from build123d import *

# Parameters (mm, degrees)
SKETCH3_W                = 76.2
SKETCH3_H                = 25.4
SKETCH3_R                = 3.175
BOSS_EXTRUDE1_DEPTH      = 2.286
BOSS_EXTRUDE1_DEPTH_BACK = 2.286


with BuildPart() as part:
    # Sketch3 → Boss-Extrude1 (new body, two sides)
    with BuildSketch(Plane.XY) as boss_extrude1_sk:
        Rectangle(SKETCH3_W, SKETCH3_H)
        with Locations((-28.575, 0)):
            Circle(SKETCH3_R, mode=Mode.SUBTRACT)
        with Locations((28.575, 0)):
            Circle(SKETCH3_R, mode=Mode.SUBTRACT)
    extrude(amount=BOSS_EXTRUDE1_DEPTH)
    extrude(boss_extrude1_sk.sketch, amount=-BOSS_EXTRUDE1_DEPTH_BACK)


solid = part.part
CAD build for the part. Positions are in the model's coordinates, mm. Round coordinates to 2 decimals unless told otherwise and drop trailing zeros. Loops run counter-clockwise (first coordinate to the right, second up) from the corner with the lowest first, then second, coordinate; pieces in that order, holes last. Notation, with made-up numbers: (18, -8.75) - (38, -8.75) arc R27 ccw to (38, 21.25) - close; hole circle Ø6 at (22.5, 38). An arc over 180 degrees is marked (long way). Put each result on its own line as item: value.
1. Two-plate mould, pull along X, no slides. Class faces 1 (the flat face through (-1, 12.7, 0)), 2 (the cylindrical face through (-31.095, -1.932, -0.032)), 3 (the flat face through (38.1, 0, 0)), 4 (the cylindrical face through (25.4, 0.1, 0)): released by +X, released by -X, zero draft, split by the parting line, or undercut.
Geometry check:
face 1: zero draft
face 2: undercut
face 3: released by +X
face 4: undercut
2. Slice it at B-B on x = 29.5. List the corners of the cut face in (y, z), and give its area (3 significant figures).
Geometry check:
outline: (-12.7, -2.29) - (-3.04, -2.29) - (-3.04, 2.29) - (-12.7, 2.29) - close; (3.04, -2.29) - (12.7, -2.29) - (12.7, 2.29) - (3.04, 2.29) - close
area: 88.4 mm²
3. Slice it at C-C on z = 0.8. List the corners of the cut face in (x, y) (3 decimals).
Geometry check:
outline: (-38.1, -12.7) - (38.1, -12.7) - (38.1, 12.7) - (-38.1, 12.7) - close; hole circle Ø6.35 at (-28.575, 0); hole circle Ø6.35 at (28.575, 0)
4. Slice it at D-D on x = -30. List the corners of the cut face in (y, z).
Geometry check:
outline: (-12.7, -2.29) - (-2.84, -2.29) - (-2.84, 2.29) - (-12.7, 2.29) - close; (2.84, -2.29) - (12.7, -2.29) - (12.7, 2.29) - (2.84, 2.29) - close
5. Slice it at A-A on y = 0. List the corners of the cut face in (x, z).
Geometry check:
outline: (-38.1, -2.29) - (-31.75, -2.29) - (-31.75, 2.29) - (-38.1, 2.29) - close; (-25.4, -2.29) - (25.4, -2.29) - (25.4, 2.29) - (-25.4, 2.29) - close; (31.75, -2.29) - (38.1, -2.29) - (38.1, 2.29) - (31.75, 2.29) - close
